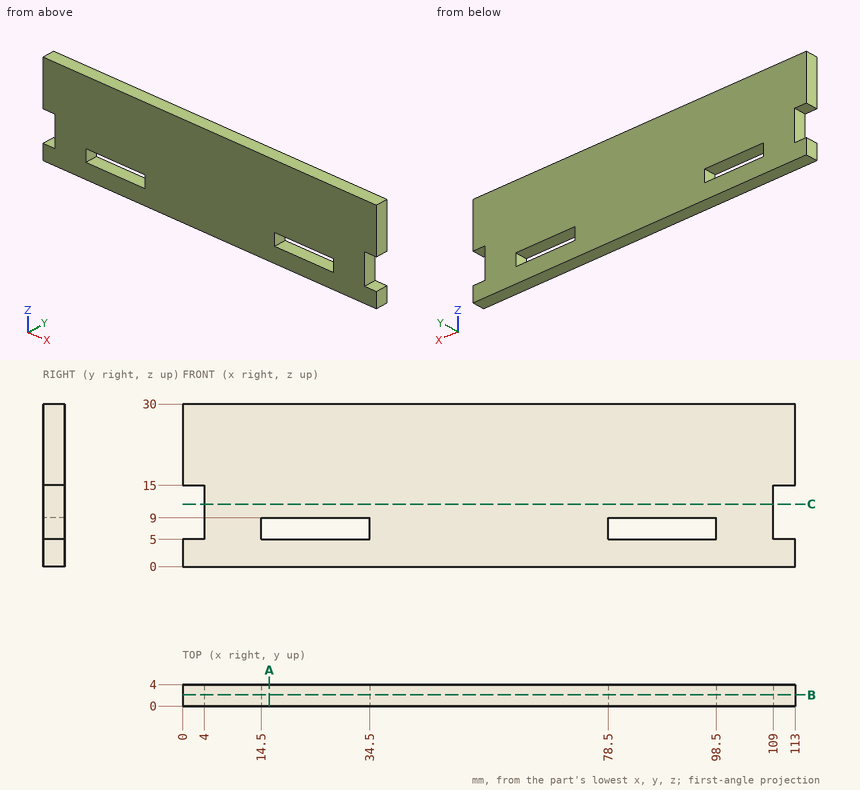
Geometry: see drawing. Coordinates: mm, zero at the bounding-box minimum. Round coordinates to 2 decimals unless told otherwise and drop trailing zeros. Loops run counter-clockwise (first coordinate to the right, second up) from the corner with the lowest first, then second, coordinate; pieces in that order, holes last.
(1) Contact query for flat-ended pins moving along their axis: pin 1 Ø1.2 at (y, z) = (2, 10) entering from +X; pin 2 Ø2 at (y, z) = (2.5, 11) entering from -X. Output: stop coordinate, or through.
From the geometry:
pin 1: stops at x = 109
pin 2: stops at x = 4
(2) Section query C-C (z = 11.5). Output: boundary loops of the cut face in (x, y).
From the geometry:
outline: (4, 0) - (109, 0) - (109, 4) - (4, 4) - close
(3) Section query B-B (y = 2.1). Output: boundary loops of the cut face in (x, z), and give its area (3 significant figures).
From the geometry:
outline: (0, 0) - (113, 0) - (113, 5) - (109, 5) - (109, 15) - (113, 15) - (113, 30) - (0, 30) - (0, 15) - (4, 15) - (4, 5) - (0, 5) - close; hole (14.5, 5) - (34.5, 5) - (34.5, 9) - (14.5, 9) - close; hole (78.5, 5) - (98.5, 5) - (98.5, 9) - (78.5, 9) - close
area: 3,150 mm2
(4) Material intervals for probe 1 along X at (y, z) = (0.35, 8); probe 2 along Z at (x, y) = (84, 1.3); probe 3 along X at (y, z) = (0.9, 14.75), sorted ascending.
From the geometry:
probe 1: x = 4 to 14.5, 34.5 to 78.5, 98.5 to 109
probe 2: z = 0 to 5, 9 to 30
probe 3: x = 4 to 109
(5) Section query A-A (x = 16). Output: boundary loops of the cut face in (y, z), and give its area (3 significant figures).
From the geometry:
outline: (0, 0) - (4, 0) - (4, 5) - (0, 5) - close; (0, 9) - (4, 9) - (4, 30) - (0, 30) - close
area: 104 mm2
